For this review, take the finished solid that the model builds, in its own axes (mm). A direction names the side the tool comes from. Give positions to 0.01 mm unless a question says otherwise; leave off trailing zeros. Order: outer loops, then holes, each group sorted by start corner. A loop starts at its lowest first (then second) coordinate and runs counter-clockwise, first axis right, second up. Notation, with made-up numbers: (28.25, 83) - (42.25, 83) arc R21 cw to (42.25, 104) - close; hole circle Ø10 at (43.25, 81). An arc over 180 degrees is marked (long way). One line per item, written item: value.
```python
from build123d import *

# Parameters (mm, degrees)
SKETCH001_R         = 20
SKETCH001_R_2       = 3.2
PAD_DEPTH           = 12
SKETCH003_W         = 30
SKETCH003_H         = 6
POCKET_DEPTH        = 6
HOLE_D              = 3.4
HOLE_DEPTH          = 25
HOLE_CBORE_D        = 4.6
HOLE_CBORE_DEPTH    = 5
HOLE001_D           = 3.4
HOLE001_DEPTH       = 10
HOLE001_CBORE_D     = 4.6
HOLE001_CBORE_DEPTH = 5
HOLE001_TIPS_R      = 1.7
HOLE002_D           = 3.4
HOLE002_DEPTH       = 10
HOLE002_CBORE_D     = 4.6
HOLE002_CBORE_DEPTH = 5
HOLE003_D           = 6.6
HOLE003_DEPTH       = 12
HOLE003_CBORE_D     = 8.5
HOLE003_CBORE_DEPTH = 6.4
FILLET002_R         = 1


with BuildPart() as part:
    # Sketch001 → Pad (new body)
    with BuildSketch(Plane.XZ):
        Polygon((30, -26.464466), (26.464466, -30), (-26.464466, -30), (-30, -26.464466), (-30, 26.464466), (-26.464466, 30), (26.464466, 30), (30, 26.464466), (30, 13), (33, 10), (33, -10), (30, -13), align=None)
        Circle(SKETCH001_R, mode=Mode.SUBTRACT)
        with Locations((-20, 20)):
            Circle(SKETCH001_R_2, mode=Mode.SUBTRACT)
        with Locations((20, 20)):
            Circle(SKETCH001_R_2, mode=Mode.SUBTRACT)
        with Locations((20, -20)):
            Circle(SKETCH001_R_2, mode=Mode.SUBTRACT)
        with Locations((-20, -20)):
            Circle(SKETCH001_R_2, mode=Mode.SUBTRACT)
    extrude(amount=PAD_DEPTH)

    # Sketch003 (on DatumPlane) → Pocket (cut)
    with BuildSketch(Plane.XZ.offset(12)):
        Polygon((24.946545, 37.208684), (9.946545, 11.227922), (4.750393, 14.227922), (19.750393, 40.208684), align=None)
        Polygon((9.946545, -11.227922), (24.946545, -37.208684), (19.750393, -40.208684), (4.750393, -14.227922), align=None)
        with Locations((-29.696938, 0)):
            Rectangle(SKETCH003_W, SKETCH003_H)
    extrude(amount=-POCKET_DEPTH, mode=Mode.SUBTRACT)

    # Hole
    with Locations(Plane.XZ.offset(6)):
        with Locations((-25, 0), (12.5, 21.650635), (12.5, -21.650635)):
            CounterBoreHole(HOLE_D / 2, HOLE_CBORE_D / 2, HOLE_CBORE_DEPTH, depth=HOLE_DEPTH)

    # Hole001
    with Locations(Plane.YZ.offset(30)):
        with Locations((-6, 20), (-6, -20)):
            CounterBoreHole(HOLE001_D / 2, HOLE001_CBORE_D / 2, HOLE001_CBORE_DEPTH, depth=HOLE001_DEPTH)

    # Hole001 tips → Hole001 tip 1 section 0
    with BuildSketch(Plane.YZ.offset(20), mode=Mode.PRIVATE) as hole001_tip_1_s0:
        with Locations((-6, 20)):
            Circle(HOLE001_TIPS_R)
    loft([hole001_tip_1_s0.sketch, Vertex(18.978537, -6, 20)], mode=Mode.SUBTRACT)

    # Hole001 tips → Hole001 tip 2 section 0
    with BuildSketch(Plane.YZ.offset(20), mode=Mode.PRIVATE) as hole001_tip_2_s0:
        with Locations((-6, -20)):
            Circle(HOLE001_TIPS_R)
    loft([hole001_tip_2_s0.sketch, Vertex(18.978537, -6, -20)], mode=Mode.SUBTRACT)

    # Hole002
    with Locations(Plane(origin=(-30, 0, 0), x_dir=(0, 1, 0), z_dir=(-1, 0, 0))):
        with Locations((-6, -20), (-6, 20)):
            CounterBoreHole(HOLE002_D / 2, HOLE002_CBORE_D / 2, HOLE002_CBORE_DEPTH, depth=HOLE002_DEPTH)

    # Hole003
    with Locations(Plane.YZ.offset(33)):
        with Locations((-6, 0)):
            CounterBoreHole(HOLE003_D / 2, HOLE003_CBORE_D / 2, HOLE003_CBORE_DEPTH, depth=HOLE003_DEPTH)

    # Fillet002
    fillet002_edges = [part.edges().sort_by_distance(p)[0] for p in [
        (-23.2, 0, -20),
        (16.8, 0, -20),
        (16.8, 0, 20),
        (-23.2, 0, 20),
    ]]
    fillet(fillet002_edges, radius=FILLET002_R)


with BuildPart() as part_1:
    # Body001 placement: moved
    add(part.part.moved(Location((0, 140, 0))))


solid = part_1.part
```
(1) Take a section at B-B (z = -25.5). Write out the cut boundary in (x, y), then the cut area to 3 significant figures.
Answers below:
outline: (-30, 128) - (11.26, 128) - (11.26, 134) - (18.19, 134) - (18.19, 128) - (30, 128) - (30, 140) - (-30, 140) - close
area: 678 mm^2
(2) Machinability: for faces 1 (the face through (24.09, 135.7, -19.93)), 2 (the face through (14, 134, -24)), 3 (the face through (10.93, 139.51, 21)), 4 (the face through (-30, 135, 0)), 5 (the face through (-25, 134, -18)), which of the approach directions +Z, -Z, +X, -X, +Y, -Y give a long, thin tool a straight path to every point of the face, cutting with its end or side? Answer none if there is none.
Answers below:
face 1: +X
face 2: -Y
face 3: +Y, -Y
face 4: +Z, -Z, -X, +Y, -Y
face 5: -X
(3) For P1, Ø5.5, axis at y = 134, z = 20, coming from the +X side; P2, Ø7.5, axis at x = -25, z = 0, coming from the -Y side; P3, Ø2, axis at y = 134, z = 20, coming from the +X side; P4, Ø6, axis at y = 134, z = 0, coming from the +X side, all flat-tipped, find the tip position at first contact; note any pin that passes through.
Answers below:
P1: stops at x = 30
P2: stops at y = 128
P3: stops at x = 16.96
P4: stops at x = 21
(4) Take a section at A-A (x = 0). Write out the cut boundary in (y, z).
Answers below:
outline: (128, -30) - (140, -30) - (140, -20) - (128, -20) - close; (128, 20) - (140, 20) - (140, 30) - (128, 30) - close
(5) Draft analysis for pull direction Z (two halves, no side actions). For faces 6 (the face through (25, 134, 18)), 7 (the face through (-13, 128, 20)), 8 (the face through (-28.257, 134.084, 28.207)), 9 (the face through (-4.336, 134.084, -19.524)), state which applies: pulls with the +Z half, pulls with the -Z half, needs draft (parallel to the pull), parting line crosses it, or undercut.
Answers below:
face 6: undercut
face 7: needs draft
face 8: pulls with the +Z half
face 9: undercut
(6) Wall thickness on line 1 (Z direction, x = -20, y = 131.5); line 2 (Z direction, x = 0, y = 131.25); line 3 (Z direction, x = 12.5, y = 139.35): over which ranges is each line inside the solid? List them lowest first. Write a range as from..to.
Answers below:
line 1: z = -30..-23.2, -16.8..-3, 3..16.8, 23.2..30
line 2: z = -30..-20, 20..30
line 3: z = -30..-23.35, -19.95..-15.61, 15.61..19.95, 23.35..30
